from build123d import *

# Parameters (mm, degrees)
BOSS_EXTRUDE1_DEPTH = 27.432
BOSS_EXTRUDE2_DEPTH = 5.08
SKETCH4_R           = 1.524
CUT_EXTRUDE1_DEPTH  = 2.286
SKETCH4_4_R         = 1.524
CUT_EXTRUDE2_DEPTH  = 43.216947178
BOSS_EXTRUDE3_DEPTH = 3.81
FILLET1_R           = 2.54
CHAMFER3_SIZE       = 1.27
CHAMFER4_SIZE       = 0.254


with BuildPart() as part:
    # Sketch1 → Boss-Extrude1 (new body)
    with BuildSketch(Plane.XY):
        Polygon((-28.575, 21.59), (-28.575, 17.78), (24.765, 17.78), (24.765, -17.78), (-28.575, -17.78), (-28.575, -21.59), (28.575, -21.59), (28.575, 21.59), align=None)
    extrude(amount=BOSS_EXTRUDE1_DEPTH)

    # Sketch1<3> → Boss-Extrude2 (add)
    with BuildSketch(Plane.XY):
        Polygon((24.765, 17.78), (-28.575, 17.78), (-28.575, 10.16), (17.145, 10.16), (17.145, -10.16), (-28.575, -10.16), (-28.575, -17.78), (24.765, -17.78), align=None)
    extrude(amount=BOSS_EXTRUDE2_DEPTH)

    # Sketch4 → Cut-Extrude1 (cut)
    # profile 1 of 4: a face of its own
    with BuildSketch(Plane.XY.offset(5.08)):
        Polygon((-20.655877438, 17.78), (-23.794122562, 17.78), (-25.363245123, 15.0622), (-23.794122562, 12.3444), (-20.655877438, 12.3444), (-19.086754877, 15.0622), align=None)
        with Locations((-22.225, 15.0622)):
            Circle(SKETCH4_R, mode=Mode.SUBTRACT)
    # profile 2 of 4: a face of its own
    with BuildSketch(Plane.XY.offset(5.08)):
        Polygon((18.714122562, 12.3444), (15.575877438, 12.3444), (14.006754877, 15.0622), (15.575877438, 17.78), (18.714122562, 17.78), (20.283245123, 15.0622), align=None)
        with Locations((17.145, 15.0622)):
            Circle(SKETCH4_R, mode=Mode.SUBTRACT)
    # profile 3 of 4: a face of its own
    with BuildSketch(Plane.XY.offset(5.08)):
        Polygon((20.283245123, -15.0622), (18.714122562, -12.3444), (15.575877438, -12.3444), (14.006754877, -15.0622), (15.575877438, -17.78), (18.714122562, -17.78), align=None)
        with Locations((17.145, -15.0622)):
            Circle(SKETCH4_R, mode=Mode.SUBTRACT)
    # profile 4 of 4: a face of its own
    with BuildSketch(Plane.XY.offset(5.08)):
        Polygon((-25.363245123, -15.0622), (-23.794122562, -12.3444), (-20.655877438, -12.3444), (-19.086754877, -15.0622), (-20.655877438, -17.78), (-23.794122562, -17.78), align=None)
        with Locations((-22.225, -15.0622)):
            Circle(SKETCH4_R, mode=Mode.SUBTRACT)
    extrude(amount=-CUT_EXTRUDE1_DEPTH, mode=Mode.SUBTRACT)

    # Sketch4<4> → Cut-Extrude2 (cut, through all)
    with BuildSketch(Plane.XY.offset(5.08)):
        with Locations((-22.225, 15.0622)):
            Circle(SKETCH4_4_R)
        with Locations((17.145, 15.0622)):
            Circle(SKETCH4_4_R)
        with Locations((-22.225, -15.0622)):
            Circle(SKETCH4_4_R)
        with Locations((17.145, -15.0622)):
            Circle(SKETCH4_4_R)
    extrude(amount=-CUT_EXTRUDE2_DEPTH, mode=Mode.SUBTRACT)

    # Sketch7 → Boss-Extrude3 (add)
    with BuildSketch(Plane.XY.offset(27.432)):
        Polygon((-28.575, 21.59), (28.575, 21.59), (28.575, -21.59), (-28.575, -21.59), (-28.575, -6.35), (-22.225, -6.35), (-22.225, 6.35), (-28.575, 6.35), align=None)
    extrude(amount=BOSS_EXTRUDE3_DEPTH)

    # Fillet1
    fillet1_edges = [part.edges().sort_by_distance(p)[0] for p in [
        (-28.575, 21.59, 15.621),
        (28.575, 21.59, 15.621),
        (28.575, -21.59, 15.621),
        (-28.575, -21.59, 15.621),
        (0, -21.59, 31.242),
        (28.575, 0, 31.242),
        (0, 21.59, 31.242),
    ]]
    fillet(fillet1_edges, radius=FILLET1_R)

    # Chamfer3
    chamfer3_edges = [part.edges().sort_by_distance(p)[0] for p in [
        (-28.575, 12.065, 27.432),
        (-28.575, 17.78, 16.256),
        (-28.575, 6.35, 29.337),
        (-28.575, -12.065, 27.432),
        (-28.575, -6.35, 29.337),
        (-25.4, 6.35, 31.242),
        (-22.225, 0, 31.242),
        (-25.4, -6.35, 31.242),
        (-28.575, -17.78, 16.256),
        (-28.575, -13.97, 5.08),
        (-28.575, 13.97, 5.08),
    ]]
    chamfer(chamfer3_edges, length=CHAMFER3_SIZE - 0.0001)  # a hair under: the kernel refuses the full size

    # Chamfer4
    chamfer4_edges = [part.edges().sort_by_distance(p)[0] for p in [
        (15.621, 15.0622, 0),
        (-23.749, -15.0622, 0),
        (15.621, -15.0622, 0),
        (-23.749, 15.0622, 0),
    ]]
    chamfer(chamfer4_edges, length=CHAMFER4_SIZE)


solid = part.part
Part model, mm, in its own coordinate system. A direction names the side the tool comes from. Round coordinates to 2 decimals unless told otherwise and drop trailing zeros. Write each loop counter-clockwise with the first axis right and the second up, starting at its lowest first coordinate (ties: lowest second). Pieces come first, ordered by that corner, then holes. Notation, with made-up numbers: M 30.5,27.25 L 62.5,27.25 A22 ccw 62.5,37.25 Z; hole C -39,80.5 d11. An arc over 180 degrees is marked long. Return JSON: item names as keys, results as strings. Group by question number.
(1) Which spindle directions (+Z, -Z, +X, -X, +Y, -Y) get a long thin tool onto all of the face, cutting with end or side? Do faces 1 (the face through (-25, -6.35, 29)), 2 (the face through (-20.77, 15.52, 1.54)), 3 (the face through (17, 12.344, 4)), 4 (the face through (-27.931, 12.611, 28.058)), 5 (the face through (-21.599, -0.107, 30.598)). Say none if no direction does.
(2) Saw through at D-D on x = 0. Write the cut outline in (y, z), then the cut area to 3 significant figures.
(3) Two-plate mould, pull along Y, no slides. Class faces 6 (the face through (27.811, -20.866, 14.15)), 7 (the face through (27.811, 20.866, 14.15)), 8 (the face through (4, 12, 5.08)): +Y half, -Y half, draft (parallel to the pull), parting line (faces both ways), or undercut.
(4) Drill centre lines: probe 1 along Y at (x, z) = (-9.5, 5); probe 2 along Y at (x, z) = (-4.5, 10); probe 3 along X at (y, z) = (14, 3.5) (3 decimals). Where is each one in solid material? Low to high.
(5) Saw through at B-B on y = 9. Write the cut outline in (x, z) (3 decimals).
(6) Pin check, flat tips, straight feed: pin 1 Ø2 at (x, y) = (-15.5, 0.5) entering from -Z; pin 2 Ø5.5 at (y, z) = (1.5, 2) entering from -X (3 decimals); pin 3 Ø3 at (y, z) = (-2, 28.5) entering from -X (3 decimals). Stop position of each tip, or through.
(7) Saw through at A-A on x = 21. Write the cut outline in (y, z), then the cut area to 3 significant figures.
Returned:
{
 "1": {"face 1": "+Z, -Z, -X", "face 2": "-Z", "face 3": "none", "face 4": "-X", "face 5": "+Z, -X"},
 "2": {"outline": "M -21.59,0 L -10.16,0 L -10.16,5.08 L -17.78,5.08 L -17.78,27.43 L 17.78,27.43 L 17.78,5.08 L 10.16,5.08 L 10.16,0 L 21.59,0 L 21.59,28.7 A2.54 ccw 19.05,31.24 L -19.05,31.24 A2.54 ccw -21.59,28.7 Z", "area": "448 mm²"},
 "3": {"face 6": "-Y half", "face 7": "+Y half", "face 8": "undercut"},
 "4": {"probe 1": "-21.59 to -10.16, 10.16 to 21.59", "probe 2": "-21.59 to -17.78, 17.78 to 21.59", "probe 3": "-28.575 to -24.75, -19.7 to 14.62, 19.67 to 28.575"},
 "5": {"outline": "M -28.575,28.702 L -27.305,27.432 L 24.765,27.432 L 24.765,5.08 L 17.145,5.08 L 17.145,0 L 28.575,0 L 28.575,28.702 A2.54 ccw 26.035,31.242 L -28.575,31.242 Z"},
 "6": {"pin 1": "z = 27.43", "pin 2": "x = 17.145", "pin 3": "x = -22.225"},
 "7": {"outline": "M -21.59,0 L 21.59,0 L 21.59,28.7 A2.54 ccw 19.05,31.24 L -19.05,31.24 A2.54 ccw -21.59,28.7 Z; hole M -17.78,5.08 L 17.78,5.08 L 17.78,27.43 L -17.78,27.43 Z", "area": "551 mm²"}
}
